from build123d import *

# Parameters (mm, degrees)
F0_W     = 29.2992349714
F0_H     = 14.8931406438
F0_R     = 6.0048631412
F0_H_2   = 4.8183426261
F1_DEPTH = 12


with BuildPart() as f1:
    # F0 (on Top) → F1 (new body)
    with BuildSketch(Plane.XY):
        with Locations((-39.1167411581, 44.4685835391)):
            Rectangle(F0_W, F0_H)
        with Locations((-38.7403294444, 43.2928875089)):
            Circle(F0_R, mode=Mode.SUBTRACT)
        with Locations((-39.1167411581, 34.6128419042)):
            Rectangle(F0_W, F0_H_2)
        Polygon((-53.7663586438, 37.0220132172), (-77.3156434298, 37.0220132172), (-77.3395821452, -40.5214428902), (0, -40.5214428902), (0, 37.0220132172), (-24.4671236724, 37.0220132172), (-24.4671236724, 32.2036705911), (-53.7663586438, 32.2036705911), align=None)
        Polygon((-67.159412581, -32.1348457524), (-67.1982951041, -23.5573574901), (-66.0232231021, -23.5573574901), (-66.0232231021, -29.1860792786), (-60.445215553, -23.52036722), (-58.9717775583, -23.52036722), (-63.3394643664, -28.2037891448), (-59.3640394509, -32.1531780064), (-61.0216520727, -32.1531780064), (-64.2655640841, -29.080113396), align=None, mode=Mode.SUBTRACT)
        Polygon((-54.3745607138, -32.0733748376), (-54.2933704932, -23.5573574901), (-53.1613752246, -23.5573574901), (-53.1613752246, -32.0733748376), align=None, mode=Mode.SUBTRACT)
        Polygon((-46.1362972856, -32.0704504848), (-47.276455909, -32.0704504848), (-47.2535975277, -23.5573574901), (-41.6997484863, -29.1860792786), (-41.6997484863, -23.5573574901), (-40.5064902602, -23.5573574901), (-40.5064902602, -32.0877228451), (-46.1362972856, -26.5450645238), align=None, mode=Mode.SUBTRACT)
        with BuildLine():
            add(Edge.make_bspline(
                [(-35.9488576651, -31.7970253527), (-33.5259176791, -32.4797704816), (-33.1114083529, -31.5621960908), (-32.6099060476, -30.5001884699)],
                knots=[0, 0, 0, 0, 3.5819525129, 3.5819525129, 3.5819525129, 3.5819525129], degree=3))
            Line((-35.9488576651, -31.7970253527), (-35.2263972163, -30.936172232))
            add(Edge.make_bspline(
                [(-33.7235666811, -30.2251502872), (-33.989623189, -31.0443080962), (-34.4412997365, -31.2153324485), (-35.2263972163, -30.936172232)],
                knots=[0, 0, 0, 0, 1.6625437809, 1.6625437809, 1.6625437809, 1.6625437809], degree=3))
            Line((-33.7235666811, -30.2251502872), (-33.7235666811, -23.5433634371))
            Line((-33.7235666811, -23.5433634371), (-32.6099060476, -23.5433634371))
            Line((-32.6099060476, -23.5433634371), (-32.6099060476, -30.5001884699))
        make_face(mode=Mode.SUBTRACT)
        Polygon((-26.5759304166, -32.1469455957), (-27.8739575297, -32.1469455957), (-23.8643418998, -23.5957931727), (-20.0629122555, -32.1894772351), (-21.3611982763, -32.1894772351), (-23.9209700376, -26.2861810625), align=None, mode=Mode.SUBTRACT)
        Polygon((-10.2736325935, -31.0030188411), (-10.2736325935, -32.1972407401), (-16.4032950997, -32.1946702898), (-12.1941762045, -24.6954783797), (-15.2269415557, -24.6954783797), (-15.2269415557, -23.5953740776), (-10.2736325935, -23.5953740776), (-14.4022190943, -31.0030188411), align=None, mode=Mode.SUBTRACT)
        with BuildLine():
            add(Edge.make_bspline(
                [(-48.1313951313, -5.793298129), (-51.9084185362, -12.8880571574), (-54.6201877296, -16.2256192416), (-62.6786500216, -21.2091294951)],
                knots=[0, 0, 0, 0, 21.1960015463, 21.1960015463, 21.1960015463, 21.1960015463], degree=3))
            Line((-62.6786500216, -21.2091294951), (-73.4323149167, -21.2091294951))
            add(Edge.make_bspline(
                [(-73.4323149167, -21.2091294951), (-57.703204453, -16.1548238248), (-48.5936999321, 0), (-49.6808459371, 19.0024100635)],
                knots=[0, 0, 0, 0, 46.7022503994, 46.7022503994, 46.7022503994, 46.7022503994], degree=3))
            Line((-49.6808459371, 19.0024100635), (-47.7940440178, 18.0804803967))
            Line((-47.7940440178, 18.0804803967), (-20.9154095501, 18.0804803967))
            Line((-20.9154095501, 18.0804803967), (-16.2641759962, 21.4805174619))
            Line((-16.2641759962, 21.4805174619), (-22.3851986229, 11.1733824015))
            Line((-22.3851986229, 11.1733824015), (-23.3154464513, 12.0788225904))
            Line((-23.3154464513, 12.0788225904), (-44.0920963883, 12.0788225904))
            add(Edge.make_bspline(
                [(-44.0920963883, 12.0788225904), (-44.2973412573, 5.6142648682), (-45.9161922336, 0.504262629), (-46.8841008842, -2.5212171022)],
                knots=[0, 0, 0, 0, 14.8646038673, 14.8646038673, 14.8646038673, 14.8646038673], degree=3))
            Line((-46.8841008842, -2.5212171022), (-31.5485745668, 8.9099174365))
            add(Edge.make_bspline(
                [(-31.5485745668, 8.9099174365), (-31.2168560922, 3.058941802), (-25.7437750697, 2.9881331138), (-20.7194462419, 5.4543670267)],
                knots=[0, 0, 0, 0, 11.3670950077, 11.3670950077, 11.3670950077, 11.3670950077], degree=3))
            Line((-20.7194462419, 5.4543670267), (-37.5409174588, -8.1352172419))
            Line((-37.5409174588, -8.1352172419), (-20.7194462419, -8.1352172419))
            Line((-20.7194462419, -8.1352172419), (-27.9845260084, -16.2464901805))
            Line((-27.9845260084, -16.2464901805), (-13.8373728842, -16.2410978228))
            add(Edge.make_bspline(
                [(-13.8373728842, -16.2410978228), (-17.871780321, -12.0312822983), (-13.6970458552, -6.6286842339), (-9.1847963631, -2.4753166363)],
                knots=[0, 0, 0, 0, 14.5307673562, 14.5307673562, 14.5307673562, 14.5307673562], degree=3))
            add(Edge.make_bspline(
                [(-9.1847963631, -2.4753166363), (-10.4274889454, -6.5475832671), (-12.3048676178, -10.4483598843), (-3.4550998826, -13.4620796889)],
                knots=[0, 0, 0, 0, 12.3910606541, 12.3910606541, 12.3910606541, 12.3910606541], degree=3))
            Line((-3.4550998826, -13.4620796889), (-9.5468144864, -21.3348828256))
            Line((-9.5468144864, -21.3348828256), (-45.1452918351, -21.172452718))
            add(Edge.make_bspline(
                [(-45.1452918351, -21.172452718), (-41.3889959455, -19.3084012717), (-37.0229622611, -17.2780938447), (-32.638940055, -11.1317606643)],
                knots=[0, 0, 0, 0, 16.0382147312, 16.0382147312, 16.0382147312, 16.0382147312], degree=3))
            Line((-32.638940055, -11.1317606643), (-46.5337000787, -11.1317606643))
            Line((-46.5337000787, -11.1317606643), (-33.2919247448, -0.691383786))
            add(Edge.make_bspline(
                [(-35.9633229673, 3.0791759491), (-35.7742495835, 2.2057159804), (-35.9496586025, 0.3463805187), (-33.2919247448, -0.691383786)],
                knots=[0, 0, 0, 0, 4.6209835727, 4.6209835727, 4.6209835727, 4.6209835727], degree=3))
            Line((-35.9633229673, 3.0791759491), (-48.1313951313, -5.793298129))
        make_face(mode=Mode.SUBTRACT)
        Polygon((-29.6582430601, 19.9509840459), (-41.5902063251, 19.9509840459), (-30.0995688885, 28.9142616093), (-24.986051023, 28.9142616093), (-31.1850644648, 23.2966467738), (-24.989714846, 23.2966467738), align=None, mode=Mode.SUBTRACT)
    extrude(amount=F1_DEPTH)


solid = f1.part
Geometry check sheet. Reference: the model listing, model coordinates, mm. A direction names the side the tool comes from. Give positions to 0.01 mm unless a question says otherwise; leave off trailing zeros. Order: outer loops, then holes, each group sorted by start corner. A loop starts at its lowest first (then second) coordinate and runs counter-clockwise, first axis right, second up.
1) Cross-section at B-B (y = 0.5). Give the number of separate pieces and of enclosed holes in the cut face, then the cut area to 3 significant figures.
Results are:
separate pieces: 4
enclosed holes: 0
area: 715 mm2
2) Cross-section at A-A (y = 46.5). Record the boundary of the cut face in (x, z).
Results are:
outline: (-53.77, 0) - (-43.82, 0) - (-43.82, 12) - (-53.77, 12) - close; (-33.66, 0) - (-24.47, 0) - (-24.47, 12) - (-33.66, 12) - close
3) Material ranges on probe 1 along Y at (x, z) = (-63, 5.75); probe 2 along X at (y, z) = (-17.5, 11); probe 3 along Y at (x, z) = (-65, 9), recorded low to high.
Results are:
probe 1: y = -40.52 to -30.28, -28.54 to -27.84, -26.12 to -21.21, -15.52 to 37.02
probe 2: x = -77.33 to -65.68, -57.29 to -38.77, -6.58 to 0
probe 3: y = -40.52 to -29.86, -28.15 to -21.21, -17.04 to 37.02
4) Tool access check on faces 4 (the flat face through (-24.3, -12.13, 5.92)), 5 (the flat face through (-39, -4, 0)). Record the directions out of +Z, -Z, +X, -X, +Y, -Y that give a thin tool (end or side, any length) a straight path to the whole face; none if there is none.
Results are:
face 4: +Z, -Z
face 5: -Z, +X, -X, +Y, -Y
5) Gauge pin test, flat ends, axial feed: pin 1 (1.3 mm diameter, centred on y = -31.5, z = 6.5, fed in from -X); pin 2 (7 mm diameter, centred on x = -38.74, y = 43.29, fed in from +Z); pin 3 (3.5 mm diameter, centred on x = -64, z = 5, fed in from +Y); pin 4 (1 mm diameter, centred on y = 39.5, z = 1.5, fed in from +X). Record the tip position at first contact, or that the pin passes through.
Results are:
pin 1: stops at x = -77.34
pin 2: passes through
pin 3: stops at y = 37.02
pin 4: stops at x = -24.47
6) Draft check along Y on faces 1 (the flat face through (-21.99, -27.83, 5.92)), 2 (the flat face through (-53.766, 45, 6)), 3 (the flat face through (-61.38, -30.15, 5.92)). Enter one of: released by +Y, released by -Y, zero draft, split by the parting line, or undercut.
Results are:
face 1: undercut
face 2: zero draft
face 3: undercut
